```python
from build123d import *

# Parameters (mm, degrees)
F0_R     = 2.032
F1_DEPTH = 2.54
F2_W     = 12.7
F2_H     = 4.064
F3_DEPTH = 10.16
F5_DEPTH = 12.7
F6_W     = 2.032
F6_H     = 7.62
F7_DEPTH = 3.81


with BuildPart() as f1:
    # F0 (on Front) → F1 (new body)
    with BuildSketch(Plane.XZ):
        Polygon((7.62, 3.81), (-7.62, 3.81), (-7.62, 2.54), (-16.51, 2.54), (-16.51, -6.35), (16.51, -6.35), (16.51, 2.54), (7.62, 2.54), align=None)
        with Locations((-12.1412, 0)):
            Circle(F0_R, mode=Mode.SUBTRACT)
        with Locations((12.1285, 0)):
            Circle(F0_R, mode=Mode.SUBTRACT)
    extrude(amount=F1_DEPTH)

    # F2 (on face) → F3 (join)
    with BuildSketch(Plane.XZ.offset(2.54)):
        with Locations((0, -4.318)):
            Rectangle(F2_W, F2_H)
    extrude(amount=F3_DEPTH)

    # F4 (on face) → F5 (join)
    with BuildSketch(Plane(origin=(-6.35, 0, 0), x_dir=(0, -1, 0), z_dir=(-1, 0, 0))):
        Polygon((8.8831661625, -2.286), (12.7, -2.286), (12.2442190351, 5.3203567963), (8.441040637, 5.0924663138), align=None)
    extrude(amount=-F5_DEPTH)

    # F6 (on face) → F7 (cut)
    with BuildSketch(Plane(origin=(0, -12.5180738926, 0.7500962617), x_dir=(1, 0, 0), z_dir=(0, -0.9982095533, 0.0598137749))):
        with Locations((0, 0.7684580196)):
            Rectangle(F6_W, F6_H)
    extrude(amount=-F7_DEPTH, mode=Mode.SUBTRACT)


solid = f1.part
```
Build history of the part. All positions in model axes, mm. A direction names the side the tool comes from. Round coordinates to 2 decimals unless told otherwise and drop trailing zeros. Write each loop counter-clockwise with the first axis right and the second up, starting at its lowest first coordinate (ties: lowest second). Pieces come first, ordered by that corner, then holes. Notation, with made-up numbers: (34.25, 78) - (44.25, 78) arc R28 cw to (44.25, 107) - close; hole circle Ø1 at (51.5, 46). An arc over 180 degrees is marked (long way). Answer as CSV lines item,"result".
Q1. Cut at D-D (x = 13.5). Write the cut outline in (y, z).
Report:
outline,"(-2.54, -6.35) - (0, -6.35) - (0, -1.5) - (-2.54, -1.5) - close; (-2.54, 1.5) - (0, 1.5) - (0, 2.54) - (-2.54, 2.54) - close"
Q2. Cut at A-A (y = -1.25). Write the cut outline in (x, z).
Report:
outline,"(-16.51, -6.35) - (16.51, -6.35) - (16.51, 2.54) - (7.62, 2.54) - (7.62, 3.81) - (-7.62, 3.81) - (-7.62, 2.54) - (-16.51, 2.54) - close; hole circle Ø4.06 at (-12.14, 0); hole circle Ø4.06 at (12.13, 0)"
Q3. Drop flat-ended pins along their axis: pin 1 (5 mm diameter, centred on y = -6.5, z = 0.5, fed in from -X); pin 2 (3 mm diameter, centred on x = -4, z = 4, fed in from -Y); pin 3 (5 mm diameter, centred on y = -10.5, z = 0, fed in from +X); pin 4 (3.5 mm diameter, centred on x = -12.14, z = 0, fed in from +Y). Give the stop position or say it passes through.
Report:
pin 1,"stops at x = -6.35"
pin 2,"stops at y = -12.41"
pin 3,"stops at x = 6.35"
pin 4,"passes through"
Q4. Pull direction X, two halves, no side cores. Call faces 1 (the flat face through (-12, -1, 2.54)), 2 (the flat face through (1.016, -11, 1)), 3 (the flat face through (-6.35, -10, -2)): +X half, -X half, draft (parallel to the pull), parting line (faces both ways), or undercut.
Report:
face 1,"draft"
face 2,"undercut"
face 3,"-X half"
Q5. Cut at C-C (x = 1.5). Write the cut outline in (y, z), and give its area (3 significant figures).
Report:
outline,"(-12.7, -6.35) - (0, -6.35) - (0, 3.81) - (-2.54, 3.81) - (-2.54, -2.29) - (-8.88, -2.29) - (-8.44, 5.09) - (-12.24, 5.32) - (-12.7, -2.29) - close"
area,"95.7 mm^2"
Q6. Drill centre lines: probe 1 along Z at (x, y) = (5, -7.25); probe 2 along X at (y, z) = (-9.5, -1); probe 3 along Y at (x, z) = (-3, 2.5). Where is each one in solid material? Low to high. Write a range as [from, to].
Report:
probe 1,"z = [-6.35, -2.29]"
probe 2,"x = [-6.35, -1.02], [1.02, 6.35]"
probe 3,"y = [-12.41, -8.6], [-2.54, 0]"
Q7. Cut at B-B (z = 3.25). Write the cut outline in (x, y).
Report:
outline,"(-7.62, -2.54) - (7.62, -2.54) - (7.62, 0) - (-7.62, 0) - close; (-6.35, -12.37) - (-1.02, -12.37) - (-1.02, -8.55) - (-6.35, -8.55) - close; (1.02, -12.37) - (6.35, -12.37) - (6.35, -8.55) - (1.02, -8.55) - close"
Q8. Tool access for faces 4 (the flat face through (0, -1, 3.81)), 5 (the flat face through (0, -10.8, -2.4)), 6 (the flat face through (-3.72, -8.66, 1.45)), 7 (the flat face through (7.62, -1, 3)), 8 (the flat face through (0, -12.7, -4)): list every direction of +Z, -Z, +X, -X, +Y, -Y with a clear straight run to the whole face (end or side of a thin tool).
Report:
face 4,"+Z, +X, -X, +Y"
face 5,"+Z"
face 6,"+X, -X"
face 7,"+Z, +X, +Y, -Y"
face 8,"+Z, -Z, +X, -X, -Y"
